from build123d import *

# Parameters (mm, degrees)
SKETCH1_R           = 60.325
BOSS_EXTRUDE1_DEPTH = 2.5
SKETCH2_R           = 4.064
CUT_EXTRUDE1_DEPTH  = 86.458827806
SKETCH8_R           = 4.1
CUT_EXTRUDE4_DEPTH  = 86.458827806


with BuildPart() as part:
    # Sketch1 → Boss-Extrude1 (new, symmetric)
    with BuildSketch(Plane(origin=(0, 0, 0), x_dir=(0, 0, -1), z_dir=(1, 0, 0))):
        Circle(SKETCH1_R)
    extrude(amount=BOSS_EXTRUDE1_DEPTH, both=True)

    # Sketch2 → Cut-Extrude1 (cut, through all)
    with BuildSketch(Plane.ZY.offset(2.5)):
        with Locations((0, 50.342959834)):
            Circle(SKETCH2_R)
        with Locations((47.879, 15.556830136)):
            Circle(SKETCH2_R)
        with Locations((29.590849347, -40.728310053)):
            Circle(SKETCH2_R)
        with Locations((-29.590849347, -40.728310053)):
            Circle(SKETCH2_R)
        with Locations((-47.879, 15.556830136)):
            Circle(SKETCH2_R)
    extrude(amount=-CUT_EXTRUDE1_DEPTH, mode=Mode.SUBTRACT)

    # Sketch8 → Cut-Extrude4 (cut, through all)
    with BuildSketch(Plane(origin=(2.5, 0, 0), x_dir=(0, 0, -1), z_dir=(1, 0, 0))):
        Circle(SKETCH8_R)
    extrude(amount=-CUT_EXTRUDE4_DEPTH, mode=Mode.SUBTRACT)


solid = part.part
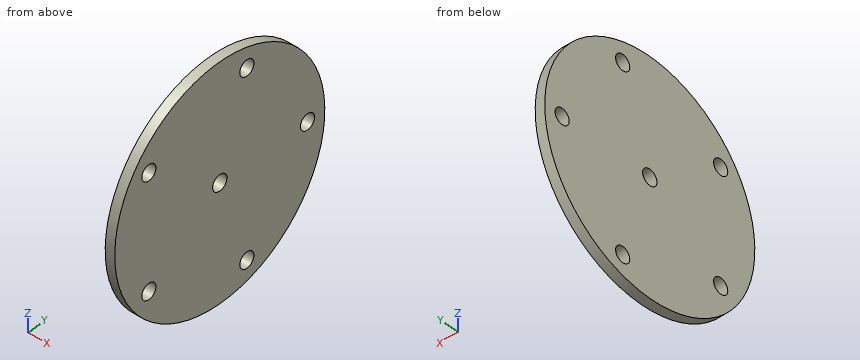
Can you work these out from the model? Positions are in its coordinate system, mm. Coordinates: 2 decimals unless noted, no trailing zeros. Loops run counter-clockwise (first coordinate to the right, second up) from the corner with the lowest first, then second, coordinate; pieces in that order, holes last. Notation, with made-up numbers: M 88,85 L 98,85 A36 ccw 98,124 Z; hole C -5.5,25.5 d5. An arc over 180 degrees is marked long. Return JSON: item names as keys, results as strings. Group by question number.
Item 1: I'm going to push flat-ended pins straight in: pin 1 Ø1.5 at (x, y) = (0, 24) entering from +Z; pin 2 Ø7.5 at (y, z) = (50.34, 0) entering from +X; pin 3 Ø3 at (x, y) = (-1.5, -44) entering from +Z; pin 4 Ø3 at (x, y) = (-1, 15) entering from +Z. Where does each tip first touch, or does it pass through?
Item 2: Imagine slicing it at C-C (y = -43). Please give me the cut outline in (x, z), and give its area (3 significant figures).
Item 3: If I drill on L1, parallel to Y at x = -0.4, z = -1; L2, parallel to Z at x = 0.1, y = 17; L3, parallel to Z at x = -0.65, y = -41.5, over which ranges is the centre line in solid material (lowest first)? Write a range as from..to.
Item 4: Imagine slicing it at A-A (z = 0). Please give me the cut outline in (x, y) (3 decimals), and give its area (3 significant figures).
Item 5: Imagine slicing it at D-D (x = 0.45). Please give me the cut outline in (y, z) (3 decimals), and give its area (3 significant figures).
Item 6: Imagine slicing it at B-B (y = 0). Please give me the cut outline in (x, z) (3 decimals), and give its area (3 significant figures).
Verdict:
{
 "1": {"pin 1": "stops at z = 55.66", "pin 2": "passes through", "pin 3": "stops at z = 42.81", "pin 4": "stops at z = 58.8"},
 "2": {"outline": "M -2.5,-42.31 L 2.5,-42.31 L 2.5,-32.96 L -2.5,-32.96 Z; M -2.5,-26.22 L 2.5,-26.22 L 2.5,26.22 L -2.5,26.22 Z; M -2.5,32.96 L 2.5,32.96 L 2.5,42.31 L -2.5,42.31 Z", "area": "356 mm^2"},
 "3": {"L1": "y = -60.32..-3.98, 3.98..46.4, 54.28..60.32", "L2": "z = -57.88..-51.68, -44.08..44.08, 51.68..57.88", "L3": "z = -43.78..-33.58, -25.6..25.6, 33.58..43.78"},
 "4": {"outline": "M -2.5,-60.325 L 2.5,-60.325 L 2.5,-4.1 L -2.5,-4.1 Z; M -2.5,4.1 L 2.5,4.1 L 2.5,46.279 L -2.5,46.279 Z; M -2.5,54.407 L 2.5,54.407 L 2.5,60.325 L -2.5,60.325 Z", "area": "522 mm^2"},
 "5": {"outline": "C 0,0 d120.65; hole C -40.728,-29.591 d8.128; hole C -40.728,29.591 d8.128; hole C 0,0 d8.2; hole C 15.557,-47.879 d8.128; hole C 15.557,47.879 d8.128; hole C 50.343,0 d8.128", "area": "11,100 mm^2"},
 "6": {"outline": "M -2.5,-60.325 L 2.5,-60.325 L 2.5,-4.1 L -2.5,-4.1 Z; M -2.5,4.1 L 2.5,4.1 L 2.5,60.325 L -2.5,60.325 Z", "area": "562 mm^2"}
}
